The listing builds one solid part. Answer for the finished solid, in the listing's coordinates (mm). A direction names the side the tool comes from. Round coordinates to 2 decimals unless told otherwise and drop trailing zeros. Write each loop counter-clockwise with the first axis right and the second up, starting at its lowest first coordinate (ties: lowest second). Pieces come first, ordered by that corner, then holes. Notation, with made-up numbers: (48.25, 26.25) - (87.25, 26.25) arc R21 cw to (87.25, 62.25) - close; hole circle Ø9 at (-19.5, -23.75). An arc over 180 degrees is marked (long way). Answer as CSV lines item,"result". Start each with the question number.
Item 1: A cutting plane is placed at B-B on x = -50.5. Determine the outline of the cut face in (y, z).
Item 2: Straight lines are drawn through the part: line 1 along Z through (x, y) = (-120, 7.25); line 2 along Z through (x, y) = (-76.5, 1.5); line 3 along Z through (x, y) = (-25, 2.75). For each, find the intervals that lie inside material, in ascending order. Write a range as [from, to].
Item 3: For a pull along Z with two mould halves and no side action, classify faces 1 (the cylindrical face through (7.493, 5.437, -0.33)), 2 (the flat face through (-105, 7, -12)), 3 (the cylindrical face through (-103.5, 2.96, 6.07)), 4 (the cylindrical face through (-107.497, 8.268, -10.687)) as pulls with the +Z half, pulls with the -Z half, needs draft (parallel to the pull), parting line crosses it, or undercut.
Item 4: A cutting plane is placed at A-A on z = 0. Determine the outline of the cut face in (x, y).
Item 5: A cutting plane is placed at C-C on y = 4.5. Determine the outline of the cut face in (x, z).
Item 6: Flat-ended cylindrical pins translate along their axes: pin 1 (1 mm diameter, centred on x = -107, y = 7.5, fed in from -Z); pin 2 (3 mm diameter, centred on x = -68, y = 3.5, fed in from -Z); pin 3 (4 mm diameter, centred on x = -106, z = -10.62, fed in from -Y). Find the tip coordinate at first contact, or state that the pin passes through.
Item 7: A cutting plane is placed at D-D on z = 5. Determine the outline of the cut face in (x, y).
Item 8: Which of the six approach directions +Z, -Z, +X, -X, +Y, -Y give full straight-line access (tool end or side, diameter ignored) to faces 5 (the flat face through (-105, 3, 0)), 6 (the flat face through (0, 9, 0)), 7 (the flat face through (-60, 3, 3.5))?
Autodesk Inventor part; units mm, degrees
ref_plane "YZ Plane" through (0, 0, 0) normal (1, 0, 0) x (0, 1, 0)
ref_plane "XZ Plane" through (0, 0, 0) normal (0, 1, 0) x (-1, 0, 0)
ref_plane "XY Plane" through (0, 0, 0) normal (0, 0, 1) x (1, 0, 0)
sketch "Boceto1" plane through (0, 0, 0) normal (0, 1, 0) x (-1, 0, 0)
  circle A0 centre (0, 0) radius 7.5
  circle A1 centre (20, 0) radius 1.75
  arc A2 (87.5, -3.5) -> (87.5, 3.5) centre (87.5, 0) ccw
  arc A3 (32.5, 3.5) -> (32.5, -3.5) centre (32.5, 0) ccw
  line L0 (100, -7.5) -> (0, -7.5)
  line L1 (100, 7.5) -> (0, 7.5)
  line L2 (87.5, -3.5) -> (32.5, -3.5)
  line L3 (87.5, 3.5) -> (32.5, 3.5)
  arc A4 (105, 2.5) -> (100, 7.5) centre (100, 2.5) ccw
  arc A5 (100, -7.5) -> (105, -2.5) centre (100, -2.5) ccw
  line L4 (105, 2.5) -> (105, -2.5)
  dimension "d0" = 15
  dimension "d3" = 3.5
  dimension "d5" = 7
  dimension "d7" = 7
  dimension "d10" = 100
  dimension "d12" = 55
  dimension "d13" = 55
extrude "Extrusión1" add sketch "Boceto1" along normal blind 9 contours A0
extrude "Extrusión2" add sketch "Boceto1" along normal blind 6 contours A0 L1 A4 L4 A5 L0
sketch "Boceto2" plane through (0, 6, 0) normal (0, 1, 0) x (1, 0, 0)
  line L0 (-100, -7.5) -> (0, -7.5)
  arc A0 (0, 7.5) -> (0, -7.5) centre (0, 0) ccw
  line L1 (0, 7.5) -> (-100, 7.5)
  arc A1 (-100, 7.5) -> (-105, 2.5) centre (-100, 2.5) ccw
  line L2 (-105, 2.5) -> (-105, -2.5)
  arc A2 (-105, -2.5) -> (-100, -7.5) centre (-100, -2.5) ccw
  line L3 (-87.5, 3.5) -> (-32.5, 3.5)
  arc A3 (-32.5, -3.5) -> (-32.5, 3.5) centre (-32.5, 0) ccw
  line L4 (-32.5, -3.5) -> (-87.5, -3.5)
  arc A4 (-87.5, 3.5) -> (-87.5, -3.5) centre (-87.5, 0) ccw
  circle A5 centre (-20, 0) radius 1.75
  arc A6 (-100, -7.5) -> (-100, 7.5) centre (-100, 0) ccw
  circle A7 centre (-120, 0) radius 1.75
  arc A8 (-120, 7.5) -> (-120, -7.5) centre (-120, 0) ccw
  line L5 (-120, -7.5) -> (-100, -7.5)
  line L6 (-120, 7.5) -> (-100, 7.5)
  dimension "d22" = 15
  dimension "d24" = 3.5
  dimension "d25" = 15
  dimension "d26" = 20
  dimension "d27" = 20
extrude "Extrusión3" add sketch "Boceto2" along normal blind 3.5 contours L5 A8 L6 A1 L2 A2 | A2 L2 A1 A6
sketch "Boceto3" plane through (0, 9.5, 0) normal (0, 1, 0) x (1, 0, 0)
  line L0 (-87.5, 3.5) -> (-32.5, 3.5)
  line L1 (-120, -7.5) -> (-100, -7.5)
  arc A0 (-100, -7.5) -> (-100, 7.5) centre (-100, 0) ccw
  line L2 (-100, 7.5) -> (-120, 7.5)
  arc A1 (-120, 7.5) -> (-120, -7.5) centre (-120, 0) ccw
  circle A2 centre (-120, 0) radius 1.75
  line L3 (0, 7.5) -> (-100, 7.5)
  line L4 (-100, 7.5) -> (-100, 10.5)
  circle A3 centre (-105.9988, 10.6207) radius 1.5
  arc A4 (-100, 10.5) -> (-111.9976, 10.5) centre (-105.9988, 10.6207) ccw
  arc A5 (-100, 7.5) -> (-105, 2.5) centre (-100, 2.5) ccw
  line L5 (-111, 7.5) -> (-100, 7.5)
  line L6 (-111.9976, 10.5) -> (-111.9976, 7.5)
  point P0 (0, 0)
  dimension "d32" = 3
  dimension "d37" = 6
  dimension "d38" = 3
  dimension "d39" = 3
extrude "Extrusión4" add sketch "Boceto3" against normal blind 2.5 contours L2 L6 A4 L4
properties part number "pieza3parte3"
Geometry says:
1,outline,"(0, -7.5) - (6, -7.5) - (6, -3.5) - (0, -3.5) - close; (0, 3.5) - (6, 3.5) - (6, 7.5) - (0, 7.5) - close"
2,line 1,"z = [-7.5, -1.75], [1.75, 7.5]"
2,line 2,"z = [-7.5, -3.5], [3.5, 7.5]"
2,line 3,"z = [-7.5, 7.5]"
3,face 1,"parting line crosses it"
3,face 2,"needs draft"
3,face 3,"pulls with the +Z half"
3,face 4,"undercut"
4,outline,"(-127.5, 6) - (-121.75, 6) - (-121.75, 9.5) - (-127.5, 9.5) - close; (-118.25, 6) - (-105, 6) - (-105, 0) - (-91, 0) - (-91, 6) - (-92.5, 6) - (-92.5, 9.5) - (-118.25, 9.5) - close; (-29, 0) - (-21.75, 0) - (-21.75, 6) - (-29, 6) - close; (-18.25, 0) - (7.5, 0) - (7.5, 9) - (-7.5, 9) - (-7.5, 6) - (-18.25, 6) - close"
5,outline,"(-105, -2.5) arc R5 ccw to (-100, -7.5) - (0, -7.5) arc R7.5 ccw to (0, 7.5) - (-100, 7.5) arc R5 ccw to (-105, 2.5) - close; hole (-87.5, -3.5) - (-32.5, -3.5) arc R3.5 ccw to (-32.5, 3.5) - (-87.5, 3.5) arc R3.5 ccw to start; hole circle Ø3.5 at (-20, 0)"
6,pin 1,"stops at z = -16.6"
6,pin 2,"stops at z = -7.5"
6,pin 3,"stops at y = 7"
7,outline,"(-125.59, 6) - (-104.33, 6) - (-104.33, 0) - (5.59, 0) - (5.59, 9) - (-5.59, 9) - (-5.59, 6) - (-94.41, 6) - (-94.41, 9.5) - (-125.59, 9.5) - close"
8,face 5,"+Z, -Z, -X, -Y"
8,face 6,"+Z, -Z, +X, +Y"
8,face 7,"+Y, -Y"
